CAD build for the part. Positions are in the model's coordinates, mm. A direction names the side the tool comes from. Round coordinates to 2 decimals unless told otherwise and drop trailing zeros. Order: outer loops, then holes, each group sorted by start corner. A loop starts at its lowest first (then second) coordinate and runs counter-clockwise, first axis right, second up. Notation, with made-up numbers: M 60.5,17 L 98.5,17 A29 cw 98.5,47 Z; hole C 23.25,42.25 d5. An arc over 180 degrees is marked long. Put each result on its own line as item: value.
```python
from build123d import *

# Parameters (mm, degrees)
F0_R     = 8.5
F1_DEPTH = 20
F3_D     = 10
F4_D     = 15
F4_DEPTH = 6
F4_TIP   = 4.5064546427
F6_D     = 1
F6_DEPTH = 10
F6_TIP   = 0.3004303095


with BuildPart() as f1:
    # F0 (on Top) → F1 (new body)
    with BuildSketch(Plane.XY):
        Circle(F0_R)
    extrude(amount=F1_DEPTH)

    # F3 (through all)
    with Locations(Plane.XY.offset(20)):
        with Locations((0, 0)):
            Hole(F3_D / 2)

    # F4
    with Locations(Plane.XY.offset(20)):
        with Locations((0, 0)):
            Hole(F4_D / 2, depth=F4_DEPTH)
            with Locations((0, 0, -(F4_DEPTH + F4_TIP / 2))):  # 118° drill point
                Cone(0, F4_D / 2, F4_TIP, mode=Mode.SUBTRACT)

    # F6
    with Locations(Plane(origin=(0, 0, 0), x_dir=(1, 0, 0), z_dir=(0, 0, -1))):
        with Locations((-6.499937755, -0.0284461158), (6.499937755, -0.0284461158)):
            Hole(F6_D / 2, depth=F6_DEPTH)
            with Locations((0, 0, -(F6_DEPTH + F6_TIP / 2))):  # 118° drill point
                Cone(0, F6_D / 2, F6_TIP, mode=Mode.SUBTRACT)


solid = f1.part
```
Item 1: Band-saw the part on B-B on z = 16.5. Give the cut face in (x, y).
Answers below:
outline: C 0,0 d17; hole C 0,0 d15
Item 2: Band-saw the part on C-C on z = 2.75. Give the cut face in (x, y).
Answers below:
outline: C 0,0 d17; hole C -6.5,0.03 d1; hole C 0,0 d10; hole C 6.5,0.03 d1
Item 3: Pin check, flat tips, straight feed: P1, Ø4, axis at y = -6, z = 10, coming from the +X side; P2, Ø4, axis at y = -4, z = 12.5, coming from the -X side; P3, Ø4, axis at y = 3.5, z = 2, coming from the +X side. Stop position of each tip, or through.
Answers below:
P1: x = 7.5
P2: x = -8.26
P3: x = 8.37
Item 4: Tool access for faces 5 (the cylindrical face through (1.08, -4.88, 6.16)), 6 (the cylindrical face through (7, 0, 5)), 7 (the cylindrical face through (7.493, 0.33, 16.958)): list every direction of +Z, -Z, +X, -X, +Y, -Y with a clear straight run to the whole face (end or side of a thin tool).
Answers below:
face 5: +Z, -Z
face 6: -Z
face 7: +Z
Item 5: Probe line 1 along Y through (x, z) = (0, 17.7); line 2 along Y through (x, z) = (0, 4.25); line 3 along X through (y, z) = (-1, 2.5). List the from-to ranges inside material, lowest first. Write a range as [from, to].
Answers below:
line 1: [-8.5, -7.5], [7.5, 8.5]
line 2: [-8.5, -5], [5, 8.5]
line 3: [-8.44, -4.9], [4.9, 8.44]
Item 6: Mould opens along X. For faces 1 (the conical face through (-6.587, 0.025, 10.248)), 2 (the cylindrical face through (-6, 0, 5)), 3 (the flat face through (0, -8, 20)), 4 (the cylindrical face through (4.57, 7.167, 9.86)) say: pulls with the +X half, pulls with the -X half, needs draft (parallel to the pull), parting line crosses it, or undercut.
Answers below:
face 1: undercut
face 2: undercut
face 3: needs draft
face 4: parting line crosses it
Item 7: Band-saw the part on A-A on x = 0. Give the cut face in (y, z).
Answers below:
outline: M -8.5,0 L -5,0 L -5,12.5 L -7.5,14 L -7.5,20 L -8.5,20 Z; M 5,0 L 8.5,0 L 8.5,20 L 7.5,20 L 7.5,14 L 5,12.5 Z
